The model under review builds one solid part; all positions refer to its coordinate system, in mm. A direction names the side the tool comes from. Round coordinates to 2 decimals unless told otherwise and drop trailing zeros. Order: outer loops, then holes, each group sorted by start corner. A loop starts at its lowest first (then second) coordinate and runs counter-clockwise, first axis right, second up.
from build123d import *

# Parameters (mm, degrees)
ESQUISSE1_R             = 1
ESQUISSE1_R_2           = 1.5
BOSS_EXTRU_1_DEPTH      = 5
ESQUISSE2_R             = 6
BOSS_EXTRU_2_DEPTH      = 3
ESQUISSE3_R             = 3.5
ENL_V_MAT_EXTRU_1_DEPTH = 5


with BuildPart() as part:
    # Esquisse1 → Boss.-Extru.1 (new body)
    with BuildSketch(Plane.XY):
        with BuildLine():
            Line((0.837209302, 7.956071932), (43.36627907, 3.48078147))
            ThreePointArc((43.36627907, 3.48078147), (46.5, 0), (43.36627907, -3.48078147))
            Line((43.36627907, -3.48078147), (0.837209302, -7.956071932))
            ThreePointArc((0.837209302, -7.956071932), (-8, 0), (0.837209302, 7.956071932))
        make_face()
        with Locations((43, 0)):
            Circle(ESQUISSE1_R, mode=Mode.SUBTRACT)
        Circle(ESQUISSE1_R_2, mode=Mode.SUBTRACT)
        with Locations((38, 0)):
            Circle(ESQUISSE1_R, mode=Mode.SUBTRACT)
        with Locations((33, 0)):
            Circle(ESQUISSE1_R, mode=Mode.SUBTRACT)
        with Locations((28, 0)):
            Circle(ESQUISSE1_R, mode=Mode.SUBTRACT)
        with Locations((23, 0)):
            Circle(ESQUISSE1_R, mode=Mode.SUBTRACT)
        with Locations((18, 0)):
            Circle(ESQUISSE1_R, mode=Mode.SUBTRACT)
        with Locations((13, 0)):
            Circle(ESQUISSE1_R, mode=Mode.SUBTRACT)
    extrude(amount=BOSS_EXTRU_1_DEPTH)

    # Esquisse2 → Boss.-Extru.2 (add)
    with BuildSketch(Plane.XY.offset(5)):
        Circle(ESQUISSE2_R)
    extrude(amount=BOSS_EXTRU_2_DEPTH)

    # Esquisse3 → Enlèv. mat.-Extru.1 (cut)
    with BuildSketch(Plane.XY.offset(8)):
        Circle(ESQUISSE3_R)
    extrude(amount=-ENL_V_MAT_EXTRU_1_DEPTH, mode=Mode.SUBTRACT)


solid = part.part
(1) We need section B-B (z = 2.5). Count the separate pieces of the cut face and the enclosed holes in it, and give its area (3 significant figures).
(2) We need section A-A (x = 13). Give the boundary of the cut face in (y, z), and give its area (3 significant figures).
(3) Tool access review of faces 1 (the cylindrical face through (27, 0, 2)), 2 (the cylindrical face through (-6, 0, 6)): name each direction out of +Z, -Z, +X, -X, +Y, -Y from which nothing blocks a thin tool from reaching the whole face with its end or side.
(4) Clearance check with flat-ended pins moving along their axes: P1, Ø1.8, axis at x = 38, y = 0, coming from the -Z side; P2, Ø1, axis at x = 7.5, z = 5, coming from the -Y side; P3, Ø5, axis at x = 20.5, y = 1.5, coming from the +Z side; P4, Ø2, axis at x = 1, y = -0.5, coming from the +Z side. State where each tip first meets the part, or that it passes through.
(5) To check wall thickness, follow L1, parallel to X at y = -0.25, z = 5.25; L2, parallel to Y at x = 0, z = 0.9; L3, parallel to Z at x = 11.5, y = 3.75. State the ranges of each line that lie inside material, in increasing order.
(6) We need section D-D (y = 2). Give the boundary of the cut face in (x, z), and give its area (3 significant figures).
(7) We need section C-C (z = 6.5). Give the boundary of the cut face in (x, y), and give its area (3 significant figures).
(8) The part is to be moulded in two halves that separate along Y. For faces 3 (the flat face through (21.8, 5.75, 2.46)), 4 (the cylindrical face through (14, 0, 2)), 5 (the flat face through (14, -2, 0)), say which applies: pulls with the +Y half, pulls with the -Y half, needs draft (parallel to the pull), parting line crosses it, or undercut.
Verdict:
1. separate pieces: 1
1. enclosed holes: 8
1. area: 588 mm2
2. outline: (-6.68, 0) - (-1, 0) - (-1, 5) - (-6.68, 5) - close; (1, 0) - (6.68, 0) - (6.68, 5) - (1, 5) - close
2. area: 56.8 mm2
3. face 1: +Z, -Z
3. face 2: +Z
4. P1: passes through
4. P2: stops at y = -7.31
4. P3: stops at z = 5
4. P4: stops at z = 3
5. L1: x = -5.99 to -3.49, 3.49 to 5.99
5. L2: y = -8 to -1.5, 1.5 to 8
5. L3: z = 0 to 5
6. outline: (-7.75, 0) - (45.87, 0) - (45.87, 5) - (5.66, 5) - (5.66, 8) - (2.87, 8) - (2.87, 3) - (-2.87, 3) - (-2.87, 8) - (-5.66, 8) - (-5.66, 5) - (-7.75, 5) - close
6. area: 273 mm2
7. outline: circle Ø12 at (0, 0); hole circle Ø7 at (0, 0)
7. area: 74.6 mm2
8. face 3: pulls with the +Y half
8. face 4: undercut
8. face 5: needs draft
